The figure shows three views and two pictorial views of one solid part (mm, origin at its lowest corner). Answer the questions. Round coordinates to 2 decimals unless told otherwise and drop trailing zeros. Loops run counter-clockwise (first coordinate to the right, second up) from the corner with the lowest first, then second, coordinate; pieces in that order, holes last. Notation, with made-up numbers: (39.25, -33) -> (82.25, -33) arc R30 cw to (82.25, -5) -> close; hole circle Ø6 at (2, 28.25). An arc over 180 degrees is marked (long way). Use a Markdown table: item, result. Add a question column.
Q1. Section B-B on z = 5.5 is taken. Give the vertices of the cut face in (x, y).
Q2. Section C-C on y = 3.65 is taken. Give the vertices of the cut face in (x, z) (1 decimal), then the cut area to 3 significant figures.
Q3. Consider line 1 (Z direction, x = 5.5, y = 2.55); line 2 (Z direction, x = 22.75, y = 0.8) (1 decimal); line 3 (X direction, y = 0.8, z = 17.75) (1 decimal). Determine where each line is inside the solid, lowest interval first.
Q4. For a pull along X with two mould halves and no side action, classify the marked faces 1 and 2 as released by +X, released by -X, zero draft, split by the parting line, or undercut.
Q5. Given pin 1 Ø2 at (x, y) = (11.5, 1) entering from -Z; pin 2 Ø1 at (y, z) = (1, 21) entering from -X, each flat-ended and moving along its own axis, determine where each tip first touches the part or whether it passes through.
Q6. Section A-A on x = 5.5 is taken. Give the vertices of the cut face in (y, z).
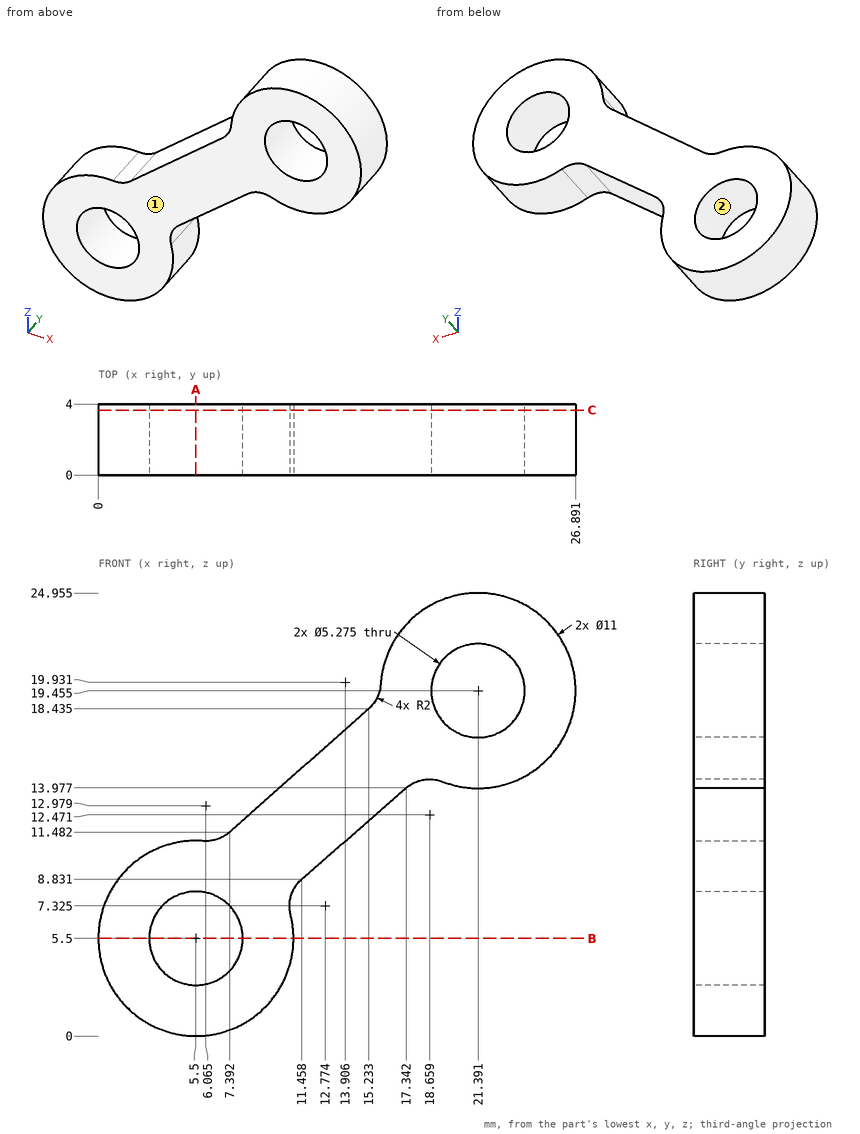
Checked values:
| question | item | result |
|---|---|---|
| 1 | outline | (0, 0) -> (2.86, 0) -> (2.86, 4) -> (0, 4) -> close; (8.14, 0) -> (11, 0) -> (11, 4) -> (8.14, 4) -> close |
| 2 | outline | (5.9, 11) arc R5.5 ccw (long way) to (10.8, 6.8) arc R2 cw to (11.5, 8.8) -> (17.3, 14) arc R2 cw to (19.4, 14.3) arc R5.5 ccw (long way) to (15.9, 19.8) arc R2 cw to (15.2, 18.4) -> (7.4, 11.5) arc R2 cw to start; hole circle Ø5.3 at (5.5, 5.5); hole circle Ø5.3 at (21.4, 19.5) |
| 2 | area | 197 mm2 |
| 3 | line 1 | z = 0 to 2.86, 8.14 to 11 |
| 3 | line 2 | z = 14.1 to 17.2, 21.7 to 24.8 |
| 3 | line 3 | x = 14.5 to 19.4, 23.4 to 26.6 |
| 4 | face 1 | zero draft |
| 4 | face 2 | undercut |
| 5 | pin 1 | stops at z = 3.21 |
| 5 | pin 2 | stops at x = 15.99 |
| 6 | outline | (0, 0) -> (4, 0) -> (4, 2.86) -> (0, 2.86) -> close; (0, 8.14) -> (4, 8.14) -> (4, 11) -> (0, 11) -> close |
